Drawing for the job (mm, zero at the part's lowest x, y, z). A direction names the side the tool comes from. Give positions to 0.01 mm unless a question says otherwise; leave off trailing zeros. Order: outer loops, then holes, each group sorted by start corner. A loop starts at its lowest first (then second) coordinate and runs counter-clockwise, first axis right, second up. Notation, with made-up numbers: (-32.5, 9) - (-28.5, 9) arc R28 ccw to (-28.5, 40) - close; hole circle Ø4 at (51, 76.25). An arc over 180 degrees is marked (long way). Use a Markdown table: item, result. Add a question column.
(1) Flat gauge pins, fed straight in: pin 1 (1.5 mm diameter, centred on y = 9, z = 10.5, fed in from -X); pin 2 (1.6 mm diameter, centred on y = 1, z = 16.5, fed in from -X); pin 3 (5 mm diameter, centred on x = 42.5, z = 16, fed in from -Y); pin 4 (6 mm diameter, centred on x = 33, y = 6.5, fed in from -Z). Where does each tip first touch, or does it go through?
(2) Slice it at B-B (x = 53.5). Write the cut outline in (y, z), then the cut area to 3 significant figures.
(3) Which spindle directions (+Z, -Z, +X, -X, +Y, -Y) get a long thin tool onto all of the face, cutting with end or side? Do the marked faces 1, 2 and 3. Say none if no direction does.
(4) Slice it at C-C (y = 7.75). Write the cut outline in (x, z), then the cut area to 3 significant figures.
(5) Wall check: line 1 (Z direction, x = 33, y = 12); line 2 (Y direction, x = 7, z = 13); line 3 (X direction, y = 6, z = 8.25). Give the ranges that are in metal, low to high.
(6) Slice it at A-A (z = 15.25). Write the cut outline in (x, y), then the cut area to 3 significant figures.
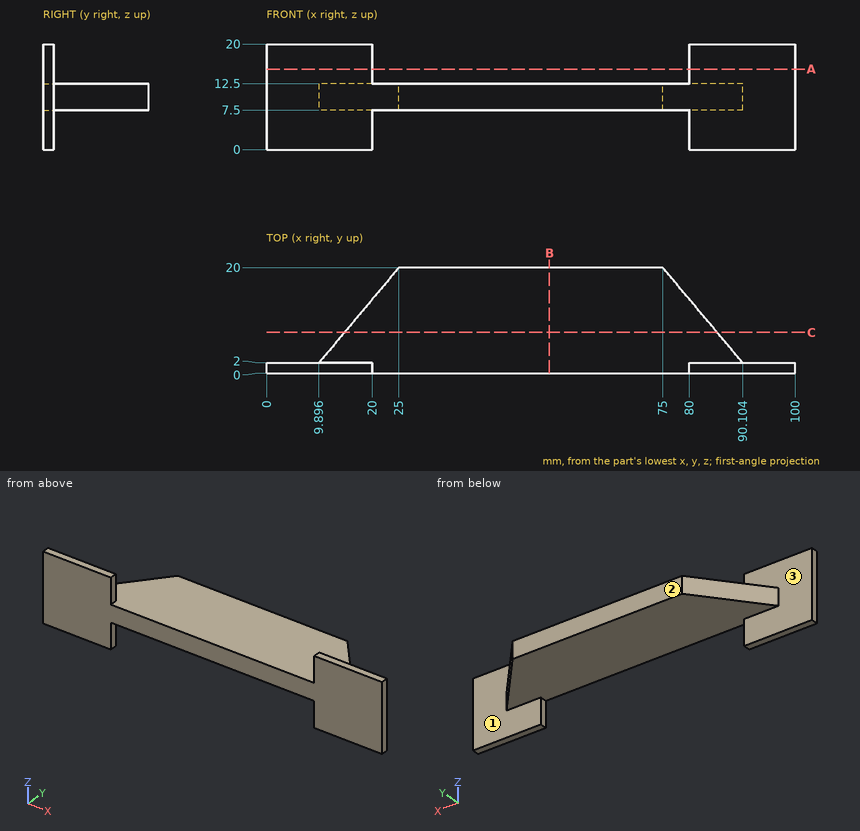
Solution:
| question | item | result |
|---|---|---|
| 1 | pin 1 | x = 15.14 |
| 1 | pin 2 | x = 0 |
| 1 | pin 3 | through |
| 1 | pin 4 | z = 7.5 |
| 2 | outline | (0, 7.5) - (20, 7.5) - (20, 12.5) - (0, 12.5) - close |
| 2 | area | 100 mm2 |
| 3 | face 1 | +X, +Y |
| 3 | face 2 | +Z, -Z, +X, -X, +Y |
| 3 | face 3 | -X, +Y |
| 4 | outline | (14.72, 7.5) - (85.28, 7.5) - (85.28, 12.5) - (14.72, 12.5) - close |
| 4 | area | 353 mm2 |
| 5 | line 1 | 7.5 to 12.5 |
| 5 | line 2 | 0 to 2 |
| 5 | line 3 | 13.25 to 86.75 |
| 6 | outline | (0, 0) - (20, 0) - (20, 2) - (0, 2) - close; (80, 0) - (100, 0) - (100, 2) - (80, 2) - close |
| 6 | area | 80.0 mm2 |
